from build123d import *

# Parameters (mm, degrees)
SKETCH1_W           = 160
SKETCH1_H           = 110
BOSS_EXTRUDE1_DEPTH = 1
SKETCH2_R           = 3
SKETCH2_R_2         = 1.5
CUT_EXTRUDE1_DEPTH  = 1


with BuildPart() as part:
    # Sketch1 → Boss-Extrude1 (new body)
    with BuildSketch(Plane(origin=(0, 0, 0), x_dir=(1, 0, 0), z_dir=(0, 1, 0))):
        Rectangle(SKETCH1_W, SKETCH1_H)
    extrude(amount=BOSS_EXTRUDE1_DEPTH)

    # Sketch2 → Cut-Extrude1 (cut)
    with BuildSketch(Plane(origin=(0, 1, 0), x_dir=(1, 0, 0), z_dir=(0, 1, 0))):
        with Locations(Location((-53, 40, 0), (0, 0, 270))):
            Circle(SKETCH2_R)
        with Locations(Location((-12.666666667, 40, 0), (0, 0, 270))):
            Circle(SKETCH2_R)
        with Locations(Location((27.666666667, 40, 0), (0, 0, 270))):
            Circle(SKETCH2_R)
        with Locations(Location((68, 40, 0), (0, 0, 270))):
            Circle(SKETCH2_R)
        with Locations(Location((-12.666666667, 0, 0), (0, 0, 270))):
            Circle(SKETCH2_R)
        with Locations(Location((27.666666667, 0, 0), (0, 0, 270))):
            Circle(SKETCH2_R)
        with Locations(Location((68, 0, 0), (0, 0, 270))):
            Circle(SKETCH2_R)
        with Locations(Location((-12.666666667, -40, 0), (0, 0, 270))):
            Circle(SKETCH2_R)
        with Locations(Location((27.666666667, -40, 0), (0, 0, 270))):
            Circle(SKETCH2_R)
        with Locations(Location((68, -40, 0), (0, 0, 270))):
            Circle(SKETCH2_R)
        with Locations(Location((-53, 0, 0), (0, 0, 270))):
            Circle(SKETCH2_R)
        with Locations(Location((-53, -40, 0), (0, 0, 270))):
            Circle(SKETCH2_R)
        with Locations(Location((-68.5, 51, 0), (0, 0, 270))):
            Circle(SKETCH2_R_2)
        with Locations(Location((-28, 51, 0), (0, 0, 270))):
            Circle(SKETCH2_R_2)
        with Locations(Location((12.5, 51, 0), (0, 0, 270))):
            Circle(SKETCH2_R_2)
        with Locations(Location((53, 51, 0), (0, 0, 270))):
            Circle(SKETCH2_R_2)
        with Locations(Location((-28, 10.5, 0), (0, 0, 270))):
            Circle(SKETCH2_R_2)
        with Locations(Location((12.5, 10.5, 0), (0, 0, 270))):
            Circle(SKETCH2_R_2)
        with Locations(Location((53, 10.5, 0), (0, 0, 270))):
            Circle(SKETCH2_R_2)
        with Locations(Location((-28, -30, 0), (0, 0, 270))):
            Circle(SKETCH2_R_2)
        with Locations(Location((12.5, -30, 0), (0, 0, 270))):
            Circle(SKETCH2_R_2)
        with Locations(Location((53, -30, 0), (0, 0, 270))):
            Circle(SKETCH2_R_2)
        with Locations(Location((-68.5, 10.5, 0), (0, 0, 270))):
            Circle(SKETCH2_R_2)
        with Locations(Location((-68.5, -30, 0), (0, 0, 270))):
            Circle(SKETCH2_R_2)
        with Locations(Location((-73, 31, 0), (0, 0, 270))):
            Circle(SKETCH2_R_2)
        with Locations(Location((-32.666666667, 31, 0), (0, 0, 270))):
            Circle(SKETCH2_R_2)
        with Locations(Location((7.666666667, 31, 0), (0, 0, 270))):
            Circle(SKETCH2_R_2)
        with Locations(Location((48, 31, 0), (0, 0, 270))):
            Circle(SKETCH2_R_2)
        with Locations(Location((-32.666666667, -9.5, 0), (0, 0, 270))):
            Circle(SKETCH2_R_2)
        with Locations(Location((7.666666667, -9.5, 0), (0, 0, 270))):
            Circle(SKETCH2_R_2)
        with Locations(Location((48, -9.5, 0), (0, 0, 270))):
            Circle(SKETCH2_R_2)
        with Locations(Location((-32.666666667, -50, 0), (0, 0, 270))):
            Circle(SKETCH2_R_2)
        with Locations(Location((7.666666667, -50, 0), (0, 0, 270))):
            Circle(SKETCH2_R_2)
        with Locations(Location((48, -50, 0), (0, 0, 270))):
            Circle(SKETCH2_R_2)
        with Locations(Location((-73, -9.5, 0), (0, 0, 270))):
            Circle(SKETCH2_R_2)
        with Locations(Location((-73, -50, 0), (0, 0, 270))):
            Circle(SKETCH2_R_2)
    extrude(amount=-CUT_EXTRUDE1_DEPTH, mode=Mode.SUBTRACT)


solid = part.part
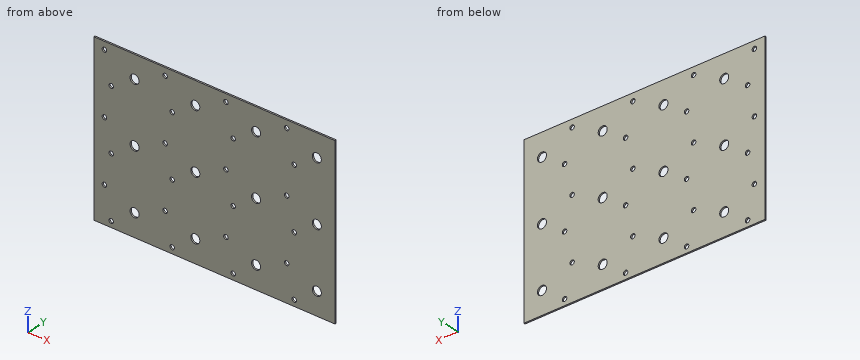
Read the model definition and answer for the solid it produces. Units are mm, in the model's axes. Coordinates: 2 decimals unless noted, no trailing zeros. Loops run counter-clockwise (first coordinate to the right, second up) from the corner with the lowest first, then second, coordinate; pieces in that order, holes last. Notation, with made-up numbers: (-37.75, 67.25) -> (-22.75, 67.25) arc R13 ccw to (-22.75, 84.25) -> close; hole circle Ø7 at (-19, 16). An arc over 180 degrees is marked (long way). Write item = value, one per line. Start each with the question number.
1) Given P1, Ø2.5, axis at x = 48, z = -31, coming from the -Y side, flat-ended and moving along its own axis, determine where the tip first touches the part or whether it passes through.
2) The part is cut by section A-A, the plane z = -40. Determine the outline of the cut face in (x, y), plus the area to 3 significant figures.
3) The part is cut by section B-B, the plane x = -53. Determine the outline of the cut face in (y, z), plus the area to 3 significant figures.
4) Find the intervals of material crossed by L1, parallel to X at y = 0.25, z = -31; L2, parallel to Z at x = 8, y = 0.65; L3, parallel to X at y = 0.75, z = -10.5, in increasing order. Write a range as from..to.
5) The part is cut by section D-D, the plane z = 39.5. Determine the outline of the cut face in (x, y), plus the area to 3 significant figures.
6) The part is cut by section C-C, the plane y = 0.7. State how many separate pieces and enclosed holes the cut face has, plus the area to 3 significant figures.
Result:
q1.P1 = through
q2.outline = (-80, 0) -> (-56, 0) -> (-56, 1) -> (-80, 1) -> close; (-50, 0) -> (-15.67, 0) -> (-15.67, 1) -> (-50, 1) -> close; (-9.67, 0) -> (24.67, 0) -> (24.67, 1) -> (-9.67, 1) -> close; (30.67, 0) -> (65, 0) -> (65, 1) -> (30.67, 1) -> close; (71, 0) -> (80, 0) -> (80, 1) -> (71, 1) -> close
q2.area = 136 mm²
q3.outline = (0, -55) -> (1, -55) -> (1, -43) -> (0, -43) -> close; (0, -37) -> (1, -37) -> (1, -3) -> (0, -3) -> close; (0, 3) -> (1, 3) -> (1, 37) -> (0, 37) -> close; (0, 43) -> (1, 43) -> (1, 55) -> (0, 55) -> close
q3.area = 92.0 mm²
q4.L1 = -80..-74.5, -71.5..-34.17, -31.17..6.17, 9.17..46.5, 49.5..80
q4.L2 = -55..-32.46, -29.54..8.04, 10.96..48.54, 51.46..55
q4.L3 = -80..-70, -67..-29.5, -26.5..11, 14..51.5, 54.5..80
q5.outline = (-80, 0) -> (-55.96, 0) -> (-55.96, 1) -> (-80, 1) -> close; (-50.04, 0) -> (-15.62, 0) -> (-15.62, 1) -> (-50.04, 1) -> close; (-9.71, 0) -> (24.71, 0) -> (24.71, 1) -> (-9.71, 1) -> close; (30.62, 0) -> (65.04, 0) -> (65.04, 1) -> (30.62, 1) -> close; (70.96, 0) -> (80, 0) -> (80, 1) -> (70.96, 1) -> close
q5.area = 136 mm²
q6.separate_pieces = 1
q6.enclosed_holes = 36
q6.area = 17,100 mm²
